The listing builds one solid part. Answer for the finished solid, in the listing's coordinates (mm). Face numbers are marked on the shaded views. A direction names the side the tool comes from. Round coordinates to 2 decimals unless told otherwise and drop trailing zeros. Write each loop counter-clockwise with the first axis right and the second up, starting at its lowest first coordinate (ties: lowest second). Pieces come first, ordered by that corner, then holes.
(1) A cutting plane is placed at C-C, the plane y = 2.75. Give the vertices of the cut face in (x, z).
(2) A cutting plane is placed at A-A, the plane z = 1.75. Give the vertices of the cut face in (x, y), and give its area (3 significant figures).
(3) A cutting plane is placed at B-B, the plane x = 3. Give the vertices of the cut face in (y, z), and give its area (3 significant figures).
(4) A cutting plane is placed at D-D, the plane y = 5.75. Give the vertices of the cut face in (x, z), and give its area (3 significant figures).
(5) The mould has two halves that part along Z. Classify the marked faces 3, 4 and 5: +Z half, -Z half, draft (parallel to the pull), parting line (faces both ways), or undercut.
(6) For the marked faces 1 and 2, determine the directions among +Z, -Z, +X, -X, +Y, -Y from which every point of the face is accessible in a straight line to the end or side of a thin tool.
(7) This flat-tipped pin is pushed along its axis until it touches: pin 1 Ø1.5 at (x, z) = (4.5, 3.5) entering from +Y. Where does it stop, or does it pass through?
(8) Find the intervals of material crossed by probe 1 along Z at (x, y) = (6.25, 0.5); probe 2 along Y at (x, z) = (3.25, 5), in increasing order.
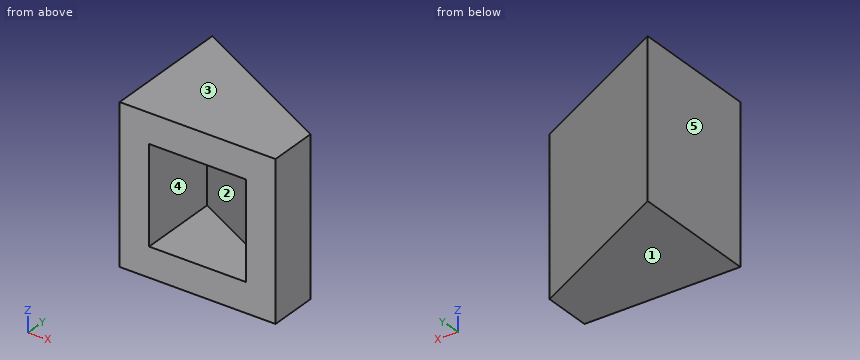
Autodesk Inventor part; units mm, degrees
ref_plane "YZ Plane" through (0, 0, 0) normal (1, 0, 0) x (0, 1, 0)
ref_plane "XZ Plane" through (0, 0, 0) normal (0, 1, 0) x (-1, 0, 0)
ref_plane "XY Plane" through (0, 0, 0) normal (0, 0, 1) x (1, 0, 0)
sketch "Sketch1" plane through (0, 0, 0) normal (0, 0, 1) x (1, 0, 0)
  line L0 (0, 0) -> (0, 6.4719)
  line L1 (0, 0) -> (7.7978, 0)
  line L2 (7.7978, 0) -> (7.7978, 2.427)
  line L3 (7.7978, 2.427) -> (0, 6.4719)
  dimension "d0" = 6.4719
  dimension "d1" = 7.7978
  dimension "d5" = 2.427
extrude "Extrusion1" add sketch "Sketch1" along normal blind 7.7978
shell "Shell1" thickness 1.4732 removed faces 1 at (5.1985, 0, 2.5993)
properties part number "Transparent Grey Peice" material "ABS Plastic"
Solutions:
1. outline: (0, 0) - (7.18, 0) - (7.18, 7.8) - (0, 7.8) - close; hole (1.47, 1.47) - (3.98, 1.47) - (3.98, 6.32) - (1.47, 6.32) - close
2. outline: (0, 0) - (1.47, 0) - (1.47, 4.05) - (6.32, 1.53) - (6.32, 0) - (7.8, 0) - (7.8, 2.43) - (0, 6.47) - close
2. area: 21.2 mm2
3. outline: (0, 0) - (4.92, 0) - (4.92, 7.8) - (0, 7.8) - (0, 6.32) - (3.26, 6.32) - (3.26, 1.47) - (0, 1.47) - close
3. area: 22.5 mm2
4. outline: (0, 0) - (1.39, 0) - (1.39, 7.8) - (0, 7.8) - close
4. area: 10.9 mm2
5. face 3: +Z half
5. face 4: undercut
5. face 5: draft
6. face 1: -Z, +X, -X, +Y, -Y
6. face 2: -Y
7. pin 1: stops at y = 4.53
8. probe 1: z = 0 to 1.47, 6.32 to 7.8
8. probe 2: y = 3.13 to 4.79
